```python
from build123d import *

# Parameters (mm, degrees)
F0_R     = 3.81
F0_R_2   = 3.683
F1_DEPTH = 5.08
F2_DEPTH = 3.683


with BuildPart() as f1:
    # F0 (on Top) → F1 (new body, symmetric)
    with BuildSketch(Plane.XY):
        Circle(F0_R)
        Circle(F0_R_2, mode=Mode.SUBTRACT)
        Circle(F0_R_2)
    extrude(amount=F1_DEPTH, both=True)

    # F0 (on Top) → F2 (cut, symmetric)
    with BuildSketch(Plane.XY):
        Circle(F0_R)
        Circle(F0_R_2, mode=Mode.SUBTRACT)
    extrude(amount=F2_DEPTH, both=True, mode=Mode.SUBTRACT)


solid = f1.part
```
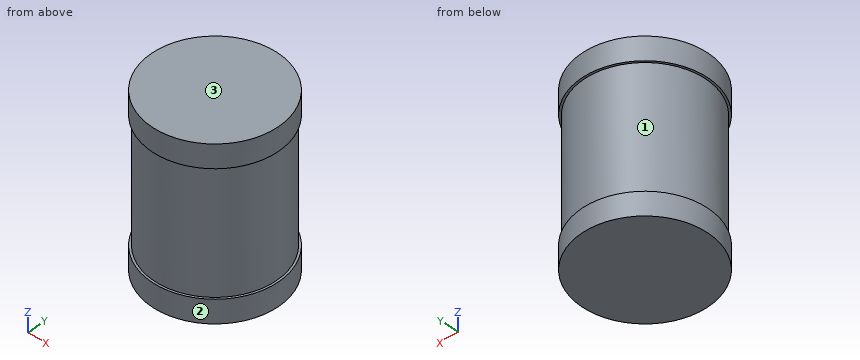
Here's how the part is built. I have some questions about the finished solid (model axes, mm). Face numbers are marked on the shaded views. Coordinates: 2 decimals unless noted, no trailing zeros. Loops run counter-clockwise (first coordinate to the right, second up) from the corner with the lowest first, then second, coordinate; pieces in that order, holes last. Notation, with made-up numbers: (83, -5) - (105, -5) arc R18 ccw to (105, 14) - close; hole circle Ø8 at (-0.5, 79). An arc over 180 degrees is marked (long way). Return JSON: item names as keys, results as strings. Group by question number.
Item 1: We'd pull the mould along Z, two halves only. Please class the marked faces 1, 2 and 3: +Z half, -Z half, draft (parallel to the pull), parting line (faces both ways), or undercut.
Item 2: If we section it at A-A on x = 0: Write out the boundary of the cut face in (y, z), and give its area (3 significant figures).
Item 3: I need wall thicknesses on line 1 (Z direction, x = -2.75, y = 2.5); line 2 (X direction, y = 2, z = -2.75); line 3 (Y direction, x = -0.75, z = 0). Which ranges of each line are inside material? Lowest first, please. Write a range as from..to.
Item 4: If we section it at C-C on z = -0.5: Write out the boundary of the cut face in (x, y).
Item 5: Will these pins go through, and if not, where does the flat tip stop? P1, Ø2, axis at y = -0.5, z = -2.5, coming from the +X side; P2, Ø2, axis at y = -2, z = -1.5, coming from the -X side; P3, Ø4, axis at x = 1.5, z = 0.5, coming from the +Y side.
Calculated:
{
 "1": {"face 1": "undercut", "face 2": "draft", "face 3": "+Z half"},
 "2": {"outline": "(-3.81, -5.08) - (3.81, -5.08) - (3.81, -3.68) - (3.68, -3.68) - (3.68, 3.68) - (3.81, 3.68) - (3.81, 5.08) - (-3.81, 5.08) - (-3.81, 3.68) - (-3.68, 3.68) - (-3.68, -3.68) - (-3.81, -3.68) - close", "area": "75.5 mm^2"},
 "3": {"line 1": "z = -5.08..-3.68, 3.68..5.08", "line 2": "x = -3.09..3.09", "line 3": "y = -3.61..3.61"},
 "4": {"outline": "circle Ø7.37 at (0, 0)"},
 "5": {"P1": "stops at x = 3.68", "P2": "stops at x = -3.54", "P3": "stops at y = 3.68"}
}
